Could you check a few things on this model? Use its own coordinates, in mm. A direction names the side the tool comes from. Give positions to 0.01 mm unless a question says otherwise; leave off trailing zeros. Order: outer loops, then holes, each group sorted by start corner. A loop starts at its lowest first (then second) coordinate and runs counter-clockwise, first axis right, second up.
(1) On a 3-axis mill with a long thin cutter (end or side, diameter ignored), from which of +Z, -Z, +X, -X, +Y, -Y can I reach the whole of each face in a straight line? I mean faces 4 (the flat face through (-18, -2, 78)), 5 (the flat face through (-66, 10, -33)), 6 (the flat face through (-12, 40, -39)). Say none if no direction works.
(2) If we mould it in two halves opening along Y, with no side actions, what happens to faces 1 (the flat face through (-76.13, -2.67, -23.17)), 2 (the flat face through (1, -50, -72)), 3 (the flat face through (-48.543, -19.93, -62.668))? For each: released by +Y, released by -Y, zero draft, split by the parting line, or undercut.
(3) Imagine slicing it at D-D, the plane z = 2.5. Write out the boundary of the cut face in (x, y).
(4) Imagine slicing it at B-B, the plane z = 80. Write out the boundary of the cut face in (x, y), then the cut area to 3 significant figures.
(5) Will these pins go through, and if not, where does the flat tip stop? pin 1 (15.5 mm diameter, centred on x = 57.5, z = -27, fed in from -Y); pin 2 (11 mm diameter, centred on y = -19.5, z = 80.5, fed in from +X); pin 3 (1.5 mm diameter, centred on x = -50, z = 23.5, fed in from +Y); pin 4 (12 mm diameter, centred on x = 69.28, z = -40, fed in from +Y).
(6) If I drill on probe 1 along Y at (x, z) = (73, -63); probe 2 along Z at (x, y) = (2.5, 21); probe 3 along X at (y, z) = (47.75, 80), over which ranges is the centre line in solid material (lowest first)?
(7) Imagine slicing it at A-A, the plane x = 0. Write out the boundary of the cut face in (y, z).
(8) Imagine slicing it at C-C, the plane y = 2. Write out the boundary of the cut face in (x, z), then the cut area to 3 significant figures.
from build123d import *

# Parameters (mm, degrees)
SKETCH6_R                                = 100
SKETCH6_R_2                              = 40
BOSS_EXTRUDE2_DEPTH                      = 50
SKETCH7_R                                = 60
CUT_EXTRUDE4_DEPTH                       = 10
SKETCH8_R                                = 60
CUT_EXTRUDE5_DEPTH                       = 70
CUT_EXTRUDE6_DEPTH                       = 101
CBORE_FOR_M12_HEX_HEAD_BOLT1_D           = 15
CBORE_FOR_M12_HEX_HEAD_BOLT1_CBORE_D     = 23.785
CBORE_FOR_M12_HEX_HEAD_BOLT1_CBORE_DEPTH = 7.5
CIRPATTERN2_COUNT                        = 3


with BuildPart() as part:
    # Sketch6 → Boss-Extrude2 (new body, symmetric)
    with BuildSketch(Plane(origin=(0, 0, 0), x_dir=(0, 0, -1), z_dir=(0, 1, 0))):
        with Locations(Location((0, 0, 0), (0, 0, 180))):  # turned: the seam where the file's is
            Circle(SKETCH6_R)
        with Locations(Location((0, 0, 0), (0, 0, 180))):  # turned: the seam where the file's is
            Circle(SKETCH6_R_2, mode=Mode.SUBTRACT)
    extrude(amount=BOSS_EXTRUDE2_DEPTH, both=True)

    # Sketch7 → Cut-Extrude4 (cut)
    with BuildSketch(Plane(origin=(0, 50, 0), x_dir=(0, 0, -1), z_dir=(0, 1, 0))):
        with Locations(Location((0, 0, 0), (0, 0, 90))):  # turned: the seam where the file's is
            Circle(SKETCH7_R)
    extrude(amount=-CUT_EXTRUDE4_DEPTH, mode=Mode.SUBTRACT)

    # Sketch8 → Cut-Extrude5 (cut)
    with BuildSketch(Plane(origin=(0, -50, 0), x_dir=(0, 0, 1), z_dir=(0, -1, 0))):
        with Locations(Location((0, 0, 0), (0, 0, 90))):  # turned: the seam where the file's is
            Circle(SKETCH8_R)
    extrude(amount=-CUT_EXTRUDE5_DEPTH, mode=Mode.SUBTRACT)

    # Sketch9 → Cut-Extrude6 (cut, through all)
    with BuildSketch(Plane(origin=(0, 0, 0), x_dir=(0, -1, 0), z_dir=(0, 0, 1))):
        Polygon((50, -18), (50, 18), (25, 18), (25, 30), (15, 30), (15, 18), (-10, 18), (-10, -18), (15, -18), (15, -30), (25, -30), (25, -18), align=None)
    cut_extrude6 = extrude(amount=CUT_EXTRUDE6_DEPTH, mode=Mode.SUBTRACT)

    # CBORE for M12 Hex Head Bolt1 (through all)
    with Locations(Plane(origin=(0, 50, 0), x_dir=(1, 0, 0), z_dir=(0, 1, 0))):
        with Locations((0, -80)):
            cbore_for_m12_hex_head_bolt1 = CounterBoreHole(CBORE_FOR_M12_HEX_HEAD_BOLT1_D / 2, CBORE_FOR_M12_HEX_HEAD_BOLT1_CBORE_D / 2, CBORE_FOR_M12_HEX_HEAD_BOLT1_CBORE_DEPTH)

    # CirPattern2: Cut-Extrude6, CBORE for M12 Hex Head Bolt1 ×3 about axis
    cirpattern2_axis = Axis((0, 0, 0), (0, 1, 0))
    add([cut_extrude6.rotate(cirpattern2_axis, i * 360 / CIRPATTERN2_COUNT) for i in range(1, CIRPATTERN2_COUNT)], mode=Mode.SUBTRACT)
    add([cbore_for_m12_hex_head_bolt1.rotate(cirpattern2_axis, i * 360 / CIRPATTERN2_COUNT) for i in range(1, CIRPATTERN2_COUNT)], mode=Mode.SUBTRACT)


solid = part.part
Answer block:
1. face 4: +Z, -Y
1. face 5: -Y
1. face 6: +Y
2. face 1: zero draft
2. face 2: released by -Y
2. face 3: undercut
3. outline: (-99.97, -50) - (-59.95, -50) - (-59.95, 20) - (-39.92, 20) - (-39.92, 40) - (-59.95, 40) - (-59.95, 50) - (-99.97, 50) - close; (39.92, 20) - (59.95, 20) - (59.95, -50) - (99.97, -50) - (99.97, 50) - (59.95, 50) - (59.95, 40) - (39.92, 40) - close
4. outline: (-60, -50) - (-18, -50) - (-18, -25) - (-30, -25) - (-30, -15) - (-18, -15) - (-18, 10) - (-7.5, 10) - (-7.5, 42.5) - (-11.89, 42.5) - (-11.89, 50) - (-60, 50) - close; (7.5, 10) - (18, 10) - (18, -15) - (30, -15) - (30, -25) - (18, -25) - (18, -50) - (60, -50) - (60, 50) - (11.89, 50) - (11.89, 42.5) - (7.5, 42.5) - close
4. area: 8,930 mm2
5. pin 1: stops at y = 10
5. pin 2: stops at x = 66.14
5. pin 3: stops at y = 40
5. pin 4: passes through
6. probe 1: y = -50 to -25, -15 to 50
6. probe 2: z = -99.97 to -39.92, 39.92 to 72.93, 87.07 to 99.97
6. probe 3: x = -60 to -11.89, 11.89 to 60
7. outline: (-50, -100) - (50, -100) - (50, -60) - (40, -60) - (40, -40) - (20, -40) - (20, -60) - (-50, -60) - close; (10, 60) - (20, 60) - (20, 40) - (40, 40) - (40, 60) - (50, 60) - (50, 68.11) - (42.5, 68.11) - (42.5, 72.5) - (10, 72.5) - close; (10, 87.5) - (42.5, 87.5) - (42.5, 91.89) - (50, 91.89) - (50, 100) - (10, 100) - close
8. outline: (-94.19, -33.59) - (-58.57, -13.03) arc R60 cw to (-18, 57.24) - (-18, 98.37) arc R100 ccw to start; (-76.19, -64.77) arc R100 ccw to (76.19, -64.77) - (40.57, -44.21) arc R60 cw to (-40.57, -44.21) - close; (18, 57.24) arc R60 cw to (58.57, -13.03) - (94.19, -33.59) arc R100 ccw to (18, 98.37) - close
8. area: 15,700 mm2
